The figure shows three views and two pictorial views of one solid part (mm, origin at its lowest corner). Answer the questions. Coordinates: 2 decimals unless noted, no trailing zeros. Write each loop counter-clockwise with the first axis right and the second up, starting at its lowest first coordinate (ties: lowest second). Pieces come first, ordered by that corner, then holes.
Item 1: Straight lines are drawn through the part: probe 1 along Y at (x, z) = (51, 4); probe 2 along X at (y, z) = (36, 2.25); probe 3 along Y at (x, z) = (6.35, 3.5) (3 decimals). For each, find the intervals that lie inside material, in ascending order.
Item 2: Section A-A (y = 19.5) is taken. Give the vertices of the cut face in (x, z), then the cut area to 3 significant figures.
Item 3: Section C-C (y = 5.08) is taken. Give the vertices of the cut face in (x, z), then the cut area to 3 significant figures.
Item 4: Determine the mould class of the marked faces 1, 2 and 3 for opening direction X: released by +X, released by -X, zero draft, split by the parting line, or undercut.
Item 5: Section D-D (z = 4.25) is taken. Give the vertices of the cut face in (x, y) (3 decimals).
Item 6: Section B-B (x = 33) is taken. Give the vertices of the cut face in (y, z).
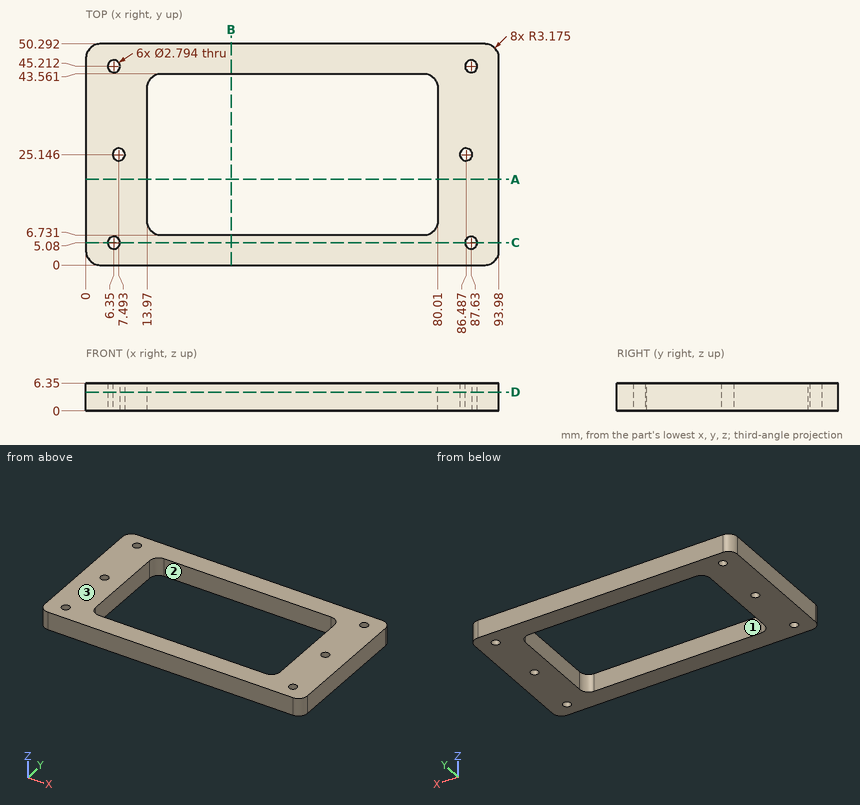
Established:
1. probe 1: y = 0 to 6.73, 43.56 to 50.29
1. probe 2: x = 0 to 13.97, 80.01 to 93.98
1. probe 3: y = 0 to 3.683, 6.477 to 24.343, 25.949 to 43.815, 46.609 to 50.292
2. outline: (0, 0) - (13.97, 0) - (13.97, 6.35) - (0, 6.35) - close; (80.01, 0) - (93.98, 0) - (93.98, 6.35) - (80.01, 6.35) - close
2. area: 177 mm2
3. outline: (0, 0) - (4.95, 0) - (4.95, 6.35) - (0, 6.35) - close; (7.75, 0) - (86.23, 0) - (86.23, 6.35) - (7.75, 6.35) - close; (89.03, 0) - (93.98, 0) - (93.98, 6.35) - (89.03, 6.35) - close
3. area: 561 mm2
4. face 1: undercut
4. face 2: undercut
4. face 3: zero draft
5. outline: (0, 3.175) arc R3.175 ccw to (3.175, 0) - (90.805, 0) arc R3.175 ccw to (93.98, 3.175) - (93.98, 47.117) arc R3.175 ccw to (90.805, 50.292) - (3.175, 50.292) arc R3.175 ccw to (0, 47.117) - close; hole circle Ø2.794 at (6.35, 5.08); hole circle Ø2.794 at (6.35, 45.212); hole circle Ø2.794 at (7.493, 25.146); hole (13.97, 9.906) arc R3.175 ccw to (17.145, 6.731) - (76.835, 6.731) arc R3.175 ccw to (80.01, 9.906) - (80.01, 40.386) arc R3.175 ccw to (76.835, 43.561) - (17.145, 43.561) arc R3.175 ccw to (13.97, 40.386) - close; hole circle Ø2.794 at (86.487, 25.146); hole circle Ø2.794 at (87.63, 5.08); hole circle Ø2.794 at (87.63, 45.212)
6. outline: (0, 0) - (6.73, 0) - (6.73, 6.35) - (0, 6.35) - close; (43.56, 0) - (50.29, 0) - (50.29, 6.35) - (43.56, 6.35) - close
